Source: CAD feature listing. Evaluate the final solid. Frame: model axes, mm. A direction names the side the tool comes from. Round coordinates to 2 decimals unless told otherwise and drop trailing zeros. Loops run counter-clockwise (first coordinate to the right, second up) from the corner with the lowest first, then second, coordinate; pieces in that order, holes last. Notation, with made-up numbers: M 31.25,76.25 L 72.25,76.25 A18 cw 72.25,107.25 Z; hole C 0.5,-11.5 d9. An arc over 180 degrees is marked long. Answer as a JSON object with one key per item and string values.
from build123d import *

# Parameters (mm, degrees)
SKETCH1_W           = 76.2
SKETCH1_H           = 57.15
BOSS_EXTRUDE1_DEPTH = 33.02
SKETCH2_R           = 5.08
BOSS_EXTRUDE2_DEPTH = 25.4
SKETCH3_W           = 1.4224
SKETCH3_H           = 6.35
BOSS_EXTRUDE3_DEPTH = 16.51


with BuildPart() as part:
    # Sketch1 → Boss-Extrude1 (new body)
    with BuildSketch(Plane(origin=(0, 0, 0), x_dir=(1, 0, 0), z_dir=(0, 1, 0))):
        Rectangle(SKETCH1_W, SKETCH1_H)
    extrude(amount=BOSS_EXTRUDE1_DEPTH)

    # Sketch2 → Boss-Extrude2 (add)
    with BuildSketch(Plane.ZY.offset(38.1)):
        with Locations((18.415, 16.51)):
            Circle(SKETCH2_R)
    extrude(amount=BOSS_EXTRUDE2_DEPTH)

    # Sketch3 → Boss-Extrude3 (add)
    with BuildSketch(Plane.XY.offset(28.575)):
        with Locations((23.1648, 16.51)):
            Rectangle(SKETCH3_W, SKETCH3_H)
        with Locations((10.3632, 16.51)):
            Rectangle(SKETCH3_W, SKETCH3_H)
    extrude(amount=BOSS_EXTRUDE3_DEPTH)


solid = part.part
Item 1: Pull-direction query (X, two-part tool) for faces 5 (the flat face through (23.876, 16, 37)), 6 (the flat face through (-38.1, 16, 0)), 7 (the flat face through (11.074, 16, 37)), 8 (the flat face through (-1, 0, 0)); classes: pulls with the +X half, pulls with the -X half, needs draft (parallel to the pull), parting line crosses it, or undercut.
Answer sheet:
{"face 5": "pulls with the +X half", "face 6": "pulls with the -X half", "face 7": "undercut", "face 8": "needs draft"}
Item 2: Section C-C on x = -6. Return the cut outline in (y, z) (3 decimals), then the cut area to 3 significant figures.
Answer sheet:
{"outline": "M 0,-28.575 L 33.02,-28.575 L 33.02,28.575 L 0,28.575 Z", "area": "1,890 mm²"}
Item 3: Section A-A on y = 16.51. Return the cut outline in (x, z) (3 decimals), then the cut area to 3 significant figures.
Answer sheet:
{"outline": "M -63.5,13.335 L -38.1,13.335 L -38.1,-28.575 L 38.1,-28.575 L 38.1,28.575 L 23.876,28.575 L 23.876,45.085 L 22.454,45.085 L 22.454,28.575 L 11.074,28.575 L 11.074,45.085 L 9.652,45.085 L 9.652,28.575 L -38.1,28.575 L -38.1,23.495 L -63.5,23.495 Z", "area": "4,660 mm²"}
Item 4: Access query for faces 1 (the cylindrical face through (-50.622, 21.547, 17.754)), 2 (the flat face through (9.652, 16, 37)), 3 (the flat face through (22.454, 16, 37)), 4 (the flat face through (-63.5, 17, 18)). Directions: +Z, -Z, +X, -X, +Y, -Y. A direction counts if a zero-diameter tool reaches every point of the face in a straight line with its end or side. Return the directions, or none.
Answer sheet:
{"face 1": "-X", "face 2": "+Z, -X, +Y, -Y", "face 3": "+Z, +Y, -Y", "face 4": "+Z, -Z, -X, +Y, -Y"}
Item 5: Contact query for flat-ended pins moving along their axis: pin 1 Ø7 at (y, z) = (17.5, 33.5) entering from -X; pin 2 Ø16.5 at (x, y) = (-8.5, 13.5) entering from +Z (3 decimals); pin 3 Ø7 at (y, z) = (15, 40) entering from +X. Output: stop coordinate, or through.
Answer sheet:
{"pin 1": "stops at x = 9.65", "pin 2": "stops at z = 28.575", "pin 3": "stops at x = 23.88"}
Item 6: Section B-B on z = -24. Return the cut outline in (x, y).
Answer sheet:
{"outline": "M -38.1,0 L 38.1,0 L 38.1,33.02 L -38.1,33.02 Z"}
Item 7: Line query: probe 1 along Z at (x, y) = (13.5, 19.5) (3 decimals); probe 2 along X at (y, z) = (9, 19.5); probe 3 along X at (y, z) = (14, 30.5). Output: solid intervals per line, ascending. Write a range as from..to.
Answer sheet:
{"probe 1": "z = -28.575..28.575", "probe 2": "x = -38.1..38.1", "probe 3": "x = 9.65..11.07, 22.45..23.88"}
